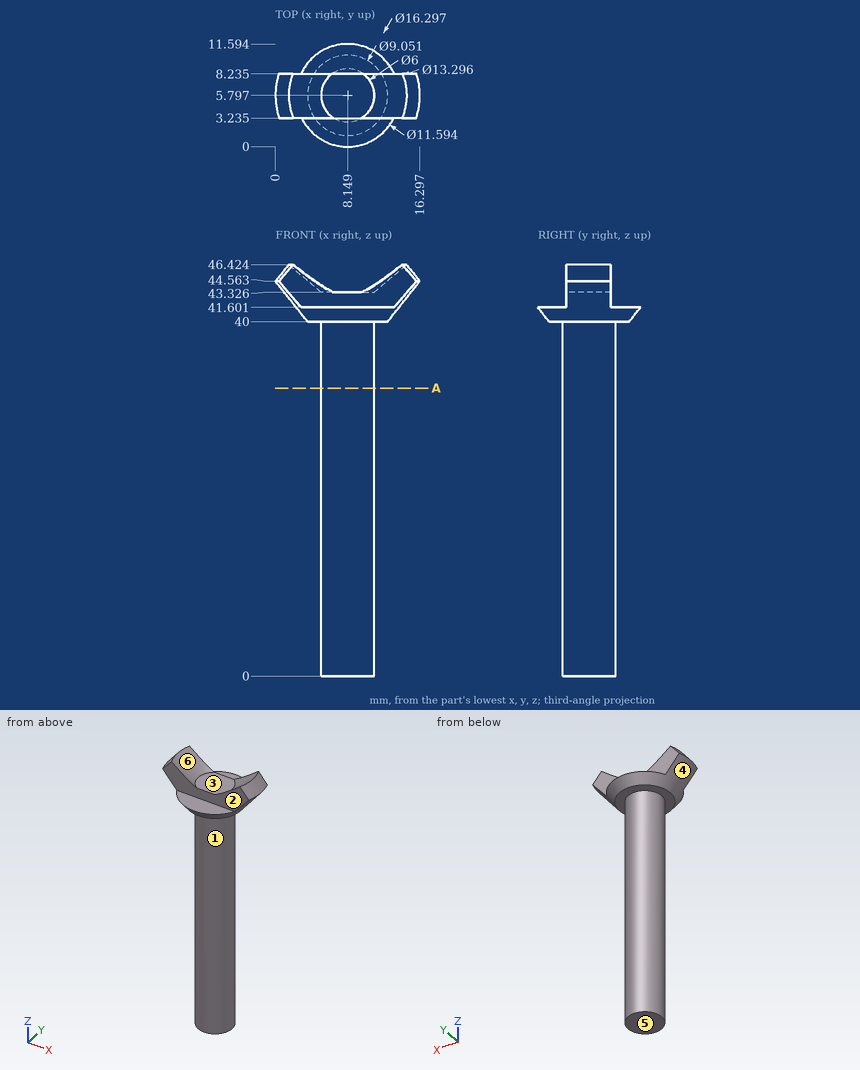
The figure shows three views and two pictorial views of one solid part (mm, origin at its lowest corner). Answer the questions. A direction names the side the tool comes from. Round coordinates to 2 decimals unless told otherwise and drop trailing zeros. Order: outer loops, then holes, each group sorted by start corner. A loop starts at its lowest first (then second) coordinate and runs counter-clockwise, first axis right, second up. Notation, with made-up numbers: M -16.5,-4 L 25.5,-4 A12 ccw 25.5,14 Z; hole C 11,39.5 d6. An arc over 180 degrees is marked long. Put each result on its own line as item: value. Start each with the question number.
Q1. A tool of negligible diameter and unlimited length cuts with its end or side. For the marked faces 1 and 2, from which of +Z, -Z, +X, -X, +Y, -Y can it reach the whole face along a straight path? Write none if from no direction.
Q2. For a pull along X with two mould halves and no side action, classify the marked faces 3, 4, 5 and 6 as pulls with the +X half, pulls with the -X half, needs draft (parallel to the pull), parting line crosses it, or undercut.
Q3. Flat-ended cylindrical pins translate along their axes: pin 1 (1.5 mm diameter, centred on x = 8.5, y = 6, fed in from +Z); pin 2 (5 mm diameter, centred on x = 10, z = 27.5, fed in from +Y); pin 3 (1.4 mm diameter, centred on x = 7, z = 43, fed in from -Y) (1 decimal). Find the tip coordinate at first contact, or state that the pin passes through.
Q4. Section A-A, the plane z = 32.5 is taken. Write down the section's boundary in (x, y), and give its area (3 significant figures).
Q5. Straight lines are drawn through the part: L1, parallel to Z at x = 6.5, y = 5.5 (1 decimal); L2, parallel to Z at x = 11.5, y = 3; L3, parallel to X at y = 7.5, z = 35. For each, find the intervals that lie inside material, in ascending order. Write a range as [from, to].
Findings below:
1. face 1: -Z
1. face 2: +Z, +X, -X, -Y
2. face 3: undercut
2. face 4: parting line crosses it
2. face 5: needs draft
2. face 6: undercut
3. pin 1: stops at z = 43.33
3. pin 2: stops at y = 8.8
3. pin 3: stops at y = 3.2
4. outline: C 8.15,5.8 d6
4. area: 28.3 mm^2
5. L1: z = [0, 43.3]
5. L2: z = [40, 41.6]
5. L3: x = [5.68, 10.62]
